```python
from build123d import *

# Parameters (mm, degrees)
BOSS_EXTRUDE1_DEPTH = 1.6
SKETCH2_R           = 5
CUT_EXTRUDE1_DEPTH  = 1.6
SKETCH3_W           = 1.6
SKETCH3_H           = 30
BOSS_EXTRUDE2_DEPTH = 200
SKETCH4_R           = 2
SKETCH4_R_2         = 3
CUT_EXTRUDE2_DEPTH  = 1032.168031188
FILLET1_R           = 10


with BuildPart() as part:
    # Sketch1 → Boss-Extrude1 (new body)
    with BuildSketch(Plane(origin=(0, 0, 0), x_dir=(1, 0, 0), z_dir=(0, 1, 0))):
        Polygon((0, 0), (576, 0), (602.078810398, 574.3), (602.078810398, 925.1), (-26.078810398, 925.1), (-26.078810398, 574.3), align=None)
    extrude(amount=BOSS_EXTRUDE1_DEPTH)

    # Sketch2 → Cut-Extrude1 (cut)
    with BuildSketch(Plane(origin=(0, 1.6, 0), x_dir=(1, 0, 0), z_dir=(0, 1, 0))):
        with Locations(Location((201.5, 115.4, 0), (0, 0, 270))):
            Circle(SKETCH2_R)
        with Locations(Location((158.5, 115.4, 0), (0, 0, 270))):
            Circle(SKETCH2_R)
    extrude(amount=-CUT_EXTRUDE1_DEPTH, mode=Mode.SUBTRACT)

    # Sketch3 → Boss-Extrude2 (add)
    with BuildSketch(Plane(origin=(0, 1.6, 0), x_dir=(1, 0, 0), z_dir=(0, 1, 0))):
        with Locations((360, 115.4)):
            Rectangle(SKETCH3_W, SKETCH3_H)
        with Locations((381.6, 115.4)):
            Rectangle(SKETCH3_W, SKETCH3_H)
    extrude(amount=BOSS_EXTRUDE2_DEPTH)

    # Sketch4 → Cut-Extrude2 (cut, through all)
    with BuildSketch(Plane(origin=(382.4, 0, 0), x_dir=(0, 0, -1), z_dir=(1, 0, 0))):
        with Locations((110.4, 191.6)):
            Circle(SKETCH4_R)
        with Locations((119.726153163, 171.6)):
            Circle(SKETCH4_R_2)
    extrude(amount=-CUT_EXTRUDE2_DEPTH, mode=Mode.SUBTRACT)

    # Fillet1
    fillet1_edges = [part.edges().sort_by_distance(p)[0] for p in [
        (360, 201.6, -130.4),
        (360, 201.6, -100.4),
        (381.6, 201.6, -130.4),
        (381.6, 201.6, -100.4),
    ]]
    fillet(fillet1_edges, radius=FILLET1_R)


solid = part.part
```
Build history of the part. All positions in model axes, mm. A direction names the side the tool comes from. Round coordinates to 2 decimals unless told otherwise and drop trailing zeros. Write each loop counter-clockwise with the first axis right and the second up, starting at its lowest first coordinate (ties: lowest second). Pieces come first, ordered by that corner, then holes.
1) 3-axis set-ups, long thin cutter, end or side, ignore diameter. For faces 1 (the flat face through (588.857, 0.789, -283.13)), 2 (the flat face through (360.8, 100, -115)): which of +Z, -Z, +X, -X, +Y, -Y reach the whole face in a straight line?
2) Drill centre lines: probe 1 along Y at (x, z) = (382, -110); probe 2 along X at (y, z) = (0.6, -115.4); probe 3 along Z at (x, y) = (381.75, 191.6). Where is each one in solid material? Low to high.
3) Pin check, flat tips, straight feed: pin 1 (6.5 mm diameter, centred on y = 191.6, z = -110.4, fed in from -X); pin 2 (1.5 mm diameter, centred on x = 107.5, z = -722, fed in from -Y); pin 3 (9 mm diameter, centred on y = 77.5, z = -117.5, fed in from +X); pin 4 (0.5 mm diameter, centred on x = 360.5, y = 60.5, fed in from +Z). Stop position of each tip, or through.
4) Mould opens along X. For faces 3 (the flat face through (380.8, 100, -115)), 4 (the flat face through (359.2, 100, -115)), 5 (the flat face through (284, 0, -469)), 6 (the flat face through (382.4, 100, -115)) say: +X half, -X half, draft (parallel to the pull), parting line (faces both ways), or undercut.
5) Band-saw the part on B-B, the plane x = 303. List the corners of the cut face in (y, z), and give its area (3 significant figures).
6) Band-saw the part on A-A, the plane y = 55. List the corners of the cut face in (x, z), and give its area (3 significant figures).
7) Band-saw the part on C-C, the plane z = -359. List the corners of the cut face in (x, y).
Ans:
1. face 1: +Z, +X, +Y, -Y
1. face 2: +Z, -Z, +Y
2. probe 1: y = 0 to 189.64, 193.56 to 201.59
2. probe 2: x = -5.24 to 153.5, 163.5 to 196.5, 206.5 to 581.24
2. probe 3: z = -130.4 to -112.4, -108.4 to -100.4
3. pin 1: stops at x = 359.2
3. pin 2: stops at y = 0
3. pin 3: stops at x = 382.4
3. pin 4: stops at z = -100.4
4. face 3: undercut
4. face 4: -X half
4. face 5: draft
4. face 6: +X half
5. outline: (0, -925.1) - (1.6, -925.1) - (1.6, 0) - (0, 0) - close
5. area: 1,480 mm2
6. outline: (359.2, -130.4) - (360.8, -130.4) - (360.8, -100.4) - (359.2, -100.4) - close; (380.8, -130.4) - (382.4, -130.4) - (382.4, -100.4) - (380.8, -100.4) - close
6. area: 96.0 mm2
7. outline: (-16.3, 0) - (592.3, 0) - (592.3, 1.6) - (-16.3, 1.6) - close
